Autodesk Inventor part; units mm, degrees
ref_plane "YZ Plane" through (0, 0, 0) normal (1, 0, 0) x (0, 1, 0)
ref_plane "XZ Plane" through (0, 0, 0) normal (0, 1, 0) x (-1, 0, 0)
ref_plane "XY Plane" through (0, 0, 0) normal (0, 0, 1) x (1, 0, 0)
sketch "Szkic1" plane through (0, 0, 0) normal (0, 0, 1) x (1, 0, 0)
  line L0 (-7.0726, 6.5674) -> (-7.0726, -23.4326)
  line L1 (-7.0726, -23.4326) -> (22.9274, -23.4326)
  line L2 (22.9274, -23.4326) -> (22.9274, -20.1326)
  line L3 (-7.0726, 6.5674) -> (-2.7726, 6.5674)
  line L4 (-2.7726, 6.5674) -> (22.9274, -20.1326)
  point P0 (0, 0)
  dimension "d0" = 30
  dimension "d1" = 30
  dimension "d2" = 3.3
  dimension "d3" = 4.3
extrude "Wyciągnięcie proste1" add sketch "Szkic1" along normal blind 20
sketch "Szkic2" plane through (22.9274, -23.4326, 0) normal (1, 0, 0) x (0, 0, -1)
  line L0 (0, 0) -> (0, 3.3)
  line L1 (0, 3.3) -> (-20, 3.3)
  line L2 (-20, 0) -> (-20, 3.3)
  line L3 (0, 0) -> (-20, 0)
  line L4 (0, 3.3) -> (0, 30)
  line L5 (0, 30) -> (-20, 30)
  line L6 (-20, 3.3) -> (-20, 30)
  line L7 (0, 3.3) -> (-20, 3.3)
  line L8 (0, 3.3) -> (-20, 3.3)
  line L9 (0, 30) -> (-20, 30)
  line L10 (-4, 3.3) -> (-16, 3.3)
  line L11 (-16, 3.3) -> (-16, 30)
  line L12 (-16, 30) -> (-4, 30)
  line L13 (-4, 30) -> (-4, 3.3)
  point P0 (0, 23.4326)
  dimension "d6" = 12
  dimension "d7" = 4
  dimension "d8" = 4
extrude "Wyciągnięcie proste2" cut sketch "Szkic2" against normal blind 25.7 contours L1 L11 L5 L13
chamfer "Faza1" distance 1.3 distance2 18.5 1 edges at (10.0774, -6.7826, 16) measured on face at (14.3607, -11.2326, 17.3333)
chamfer "Faza2" distance 1.3 distance2 18.5 1 edges at (10.0774, -6.7826, 4) measured on face at (5.7941, -2.3326, 2.6667)
fillet "Zaokrąglenie1" radius 0.8 4 edges at (10.0774, -6.7826, 17.3) (10.0774, -6.7826, 2.7) (10.0774, -6.7826, 20) (10.0774, -6.7826, 0)
fillet "Zaokrąglenie2" radius 0.8 2 edges at (22.9274, -20.1326, 10) (-2.7726, 6.5674, 10)
sketch "Szkic3" plane through (-7.0726, -23.4326, 0) normal (0, -1, 0) x (1, 0, 0)
  line L0 (0, 0) -> (30, 0)
  line L1 (30, 0) -> (30, 20)
  line L2 (0, 20) -> (30, 20)
  line L3 (0, 0) -> (0, 20)
  point P0 (7.0726, 0)
  point P1 (18.05, 10)
  dimension "d19" = 11.95
hole "Otwór1" at (10.9774, -23.4326, 10) direction (0, 1, 0) diameter 5.3 end through all
sketch "Szkic4" plane through (-7.0726, -23.4326, 0) normal (-1, 0, 0) x (0, 0, 1)
  line L0 (0, 30) -> (0, 0)
  line L1 (0, 0) -> (20, 0)
  line L2 (20, 30) -> (20, 0)
  line L3 (0, 30) -> (20, 30)
  point P0 (0, 23.4326)
  point P1 (10, 18.05)
  dimension "d27" = 11.95
hole "Otwór2" at (-7.0726, -5.3826, 10) direction (1, 0, 0) diameter 5.3 end through all
properties part number "COTS_GENERIC_20x20mm_Angle_Bracket" material "Stal nierdzewna 440C"
Design review of the part built by this model. Coordinates are the model's own, in mm. A direction names the side the tool comes from. Round coordinates to 2 decimals unless told otherwise and drop trailing zeros. Write each loop counter-clockwise with the first axis right and the second up, starting at its lowest first coordinate (ties: lowest second). Pieces come first, ordered by that corner, then holes. Notation, with made-up numbers: (-40, -22) - (18, -22) arc R28 cw to (18, -4) - close; hole circle Ø1 at (81, 58.25). An arc over 180 degrees is marked (long way). Return JSON: item names as keys, results as strings. Group by question number.
Item 1: Insertion check: P1, Ø11.5, axis at x = 10, z = 9.5, coming from the +Y side; P2, Ø1.5, axis at x = 9.5, y = -9.5, coming from the -Z side; P3, Ø10, axis at x = 19.5, z = 3, coming from the +Y side. Each pin has a flat end and moves straight along its axis. Give the tip position at first contact, or say it passes through.
Item 2: For probe 1 along X at (y, z) = (-22.7, 10); probe 2 along Y at (x, z) = (-5.65, 10); probe 3 along X at (y, z) = (-14.5, 14), list the stretches that pass through material, from the lowest coordinate up. Write a range as [from, to].
Item 3: We need section B-B on z = 8. Write out the cut boundary in (x, y).
Item 4: The part is to be moulded in two halves that separate along Z. For faces 3 (the face through (-7.073, -8.2, 9.9)), 4 (the face through (9.741, -6.751, 2.506)), 5 (the face through (9.75, -6.77, 0.24)), 6 (the face through (10, -20.133, 13)), say which applies: pulls with the +Z half, pulls with the -Z half, needs draft (parallel to the pull), parting line crosses it, or undercut.
Item 5: Machinability: for faces 1 (the face through (5.745, -10.646, 16.892)), 2 (the face through (4, -12, 0)), which of the approach directions +Z, -Z, +X, -X, +Y, -Y give a long, thin tool a straight path to every point of the face, cutting with its end or side? Answer none if there is none.
Item 6: We need section A-A on z = 10. Write out the cut boundary in (x, y).
Model answer:
{
 "1": {"P1": "stops at y = -20.13", "P2": "stops at z = 0", "P3": "stops at y = -11.48"},
 "2": {"probe 1": "x = [-7.07, 8.33], [13.63, 22.93]", "probe 2": "y = [-23.43, -8.03], [-2.73, 6.57]", "probe 3": "x = [-7.07, -2.77]"},
 "3": {"outline": "(-7.07, -23.43) - (9.24, -23.43) - (9.24, -20.13) - (-2.77, -20.13) - (-2.77, -7.12) - (-7.07, -7.12) - close; (-7.07, -3.64) - (-2.77, -3.64) - (-2.77, 5.77) arc R0.8 ccw to (-3.57, 6.57) - (-7.07, 6.57) - close; (12.72, -23.43) - (22.93, -23.43) - (22.93, -20.93) arc R0.8 ccw to (22.13, -20.13) - (12.72, -20.13) - close"},
 "4": {"face 3": "needs draft", "face 4": "undercut", "face 5": "pulls with the -Z half", "face 6": "undercut"},
 "5": {"face 1": "+X, +Y", "face 2": "-Z, +X, -X, +Y, -Y"},
 "6": {"outline": "(-7.07, -23.43) - (8.33, -23.43) - (8.33, -20.13) - (-2.77, -20.13) - (-2.77, -8.03) - (-7.07, -8.03) - close; (-7.07, -2.73) - (-2.77, -2.73) - (-2.77, 5.77) arc R0.8 ccw to (-3.57, 6.57) - (-7.07, 6.57) - close; (13.63, -23.43) - (22.93, -23.43) - (22.93, -20.93) arc R0.8 ccw to (22.13, -20.13) - (13.63, -20.13) - close"}
}
